Autodesk Inventor part; units mm, degrees
ref_plane "YZ Plane" through (0, 0, 0) normal (1, 0, 0) x (0, 1, 0)
ref_plane "XZ Plane" through (0, 0, 0) normal (0, 1, 0) x (-1, 0, 0)
ref_plane "XY Plane" through (0, 0, 0) normal (0, 0, 1) x (1, 0, 0)
sketch "Boceto1" plane through (0, 0, 0) normal (0, 0, 1) x (1, 0, 0)
  circle A0 centre (0, 0) radius 185
  circle A1 centre (0, 0) radius 183.8
  dimension "d0" = 370
  dimension "d1" = 367.6
extrude "Extrusión1" add sketch "Boceto1" along normal blind 1.2 contours A1
extrude "Extrusión2" add sketch "Boceto1" along normal blind 21.2
fillet "Empalme1" radius 2 1 edges at (-183.8, 0, 1.2)
sketch "Boceto2" plane through (0, 0, 1.2) normal (0, 0, 1) x (1, 0, 0)
  circle A0 centre (0, 0) radius 20
  dimension "d7" = 40
extrude "Extrusión3" cut sketch "Boceto2" against normal blind 10
properties part number "tapa_tambor"
Can you work these out from the model? Positions are in its coordinate system, mm. A direction names the side the tool comes from. Round coordinates to 2 decimals unless told otherwise and drop trailing zeros. Loops run counter-clockwise (first coordinate to the right, second up) from the corner with the lowest first, then second, coordinate; pieces in that order, holes last. Notation, with made-up numbers: (57, 73) - (62, 73) arc R22 cw to (62, 94) - close; hole circle Ø11 at (-6, 30). An arc over 180 degrees is marked (long way). Answer in a Markdown table with one row per item. Add a question column.
Q1. For pin 1 Ø6 at (x, z) = (-133, 11) entering from +Y; pin 2 Ø2 at (x, z) = (84.5, 18.5) entering from +Y; pin 3 Ø8 at (y, z) = (-120, 17) entering from +X; pin 4 Ø3 at (x, y) = (-38, 47) entering from -Z, each with a flat end and sliding along its axis, tell me the tip position at first contact or that it passes through.
Q2. Which directions (+Z, -Z, +X, -X, +Y, -Y) give clear straight access to the entire face, cutting with the end or side of a thin tool? Please do faces 1 (the cylindrical face through (-4.336, -19.524, 0.608)), 2 (the cylindrical face through (-39.84, 179.43, 12.07)).
Q3. I want a section at A-A on x = 0. List the corners of the cut face in (y, z) for me.
Q4. We'd pull the mould along Y, two halves only. Please class faces 3 (the flat face through (-3, -38, 1.2)), 4 (the flat face through (-3, -39, 0)), 5 (the cylindrical face through (99.455, -155.993, 10.452)): pulls with the +Y half, pulls with the -Y half, needs draft (parallel to the pull), parting line crosses it, or undercut.
Q5. I need wall thicknesses on L1, parallel to Y at x = 0, z = 13.5; L2, parallel to Y at x = 0, z = 0.65; L3, parallel to Z at x = 38.5, y = -158. Which ranges of each line are inside material? Lowest first, please.
Q6. I want a section at C-C on z = 11. List the corners of the cut face in (x, y) for me, and give its area (3 significant figures).
A:
| question | item | result |
|---|---|---|
| 1 | pin 1 | y = 131.62 |
| 1 | pin 2 | y = 165.08 |
| 1 | pin 3 | x = 144.11 |
| 1 | pin 4 | z = 0 |
| 2 | face 1 | +Z, -Z |
| 2 | face 2 | +Z |
| 3 | outline | (-185, 0) - (-20, 0) - (-20, 1.2) - (-181.8, 1.2) arc R2 cw to (-183.8, 3.2) - (-183.8, 21.2) - (-185, 21.2) - close; (20, 0) - (185, 0) - (185, 21.2) - (183.8, 21.2) - (183.8, 3.2) arc R2 cw to (181.8, 1.2) - (20, 1.2) - close |
| 4 | face 3 | undercut |
| 4 | face 4 | needs draft |
| 4 | face 5 | parting line crosses it |
| 5 | L1 | -185 to -183.8, 183.8 to 185 |
| 5 | L2 | -185 to -20, 20 to 185 |
| 5 | L3 | 0 to 1.2 |
| 6 | outline | circle Ø370 at (0, 0); hole circle Ø367.6 at (0, 0) |
| 6 | area | 1,390 mm^2 |
